from build123d import *

# Parameters (mm, degrees)
BOSS_EXTRUDE1_DEPTH     = 25.4
CUT_EXTRUDE1_DEPTH      = 58.783799795
CUT_EXTRUDE1_DEPTH_BACK = 58.783799795
SKETCH2_R               = 6.35


with BuildPart() as part:
    # Sketch1 → Boss-Extrude1 (new, symmetric)
    with BuildSketch(Plane.XY):
        Polygon((-25.4, 0), (25.4, 0), (32.118057965, 38.1), (35.244822581, 37.548667036), (28.064141329, -3.175), (-28.064141329, -3.175), (-35.244822581, 37.548667036), (-32.118057965, 38.1), align=None)
    extrude(amount=BOSS_EXTRUDE1_DEPTH, both=True)

    # Sketch2 → Cut-Extrude1 (cut, two sides: drawn at the far end of the back side and taken through both)
    with BuildSketch(Plane(origin=(0, 0, 0), x_dir=(0, 0, -1), z_dir=(1, 0, 0)).offset(-CUT_EXTRUDE1_DEPTH_BACK)):
        with Locations(Location((0, 25.4, 0), (0, 0, 90))):
            Circle(SKETCH2_R)
    extrude(amount=CUT_EXTRUDE1_DEPTH + CUT_EXTRUDE1_DEPTH_BACK, mode=Mode.SUBTRACT)


solid = part.part
Source: CAD feature listing. Evaluate the final solid. Frame: model axes, mm. A direction names the side the tool comes from. Give positions to 0.01 mm unless a question says otherwise; leave off trailing zeros. Write each loop counter-clockwise with the first axis right and the second up, starting at its lowest first coordinate (ties: lowest second). Pieces come first, ordered by that corner, then holes. Notation, with made-up numbers: M 81.5,-6 L 125.5,-6 A17 ccw 125.5,23 Z; hole C 29,39.25 d1. An arc over 180 degrees is marked long. Answer as a JSON object with one key per item and string values.
Q1. Contact query for flat-ended pins moving along their axis: P1, Ø5, axis at y = 11, z = 13.5, coming from the -X side; P2, Ø1, axis at y = 22, z = -10.5, coming from the +X side; P3, Ø16.5, axis at y = 25.4, z = 0, coming from the +X side. Output: stop coordinate, or through.
Geometry check:
{"P1": "stops at x = -31", "P2": "stops at x = 32.59", "P3": "stops at x = 34.56"}
Q2. Cut plane D-D, the plane y = 15. Return the cut outline in (x, z).
Geometry check:
{"outline": "M -31.27,-25.4 L -28.04,-25.4 L -28.04,25.4 L -31.27,25.4 Z; M 28.04,-25.4 L 31.27,-25.4 L 31.27,25.4 L 28.04,25.4 Z"}
Q3. Cut plane C-C, the plane z = 0. Return the cut outline in (x, y) (3 decimals).
Geometry check:
{"outline": "M -35.245,37.549 L -34.222,31.75 L -30.998,31.75 L -32.118,38.1 Z; M -31.983,19.05 L -28.064,-3.175 L 28.064,-3.175 L 31.983,19.05 L 28.759,19.05 L 25.4,0 L -25.4,0 L -28.759,19.05 Z; M 30.998,31.75 L 34.222,31.75 L 35.245,37.549 L 32.118,38.1 Z"}
Q4. Cut plane A-A, the plane z = 9. Return the cut outline in (x, y) (3 decimals), then the cut area to 3 significant figures.
Geometry check:
{"outline": "M -35.245,37.549 L -28.064,-3.175 L 28.064,-3.175 L 35.245,37.549 L 32.118,38.1 L 25.4,0 L -25.4,0 L -32.118,38.1 Z", "area": "424 mm^2"}
Q5. Access query for faces 4 (the face through (0, -1, -25.4)), 5 (the face through (-28.06, 15.08, 0.36)). Directions: +Z, -Z, +X, -X, +Y, -Y. A direction counts if a zero-diameter tool reaches every point of the face in a straight line with its end or side. Return the directions, or none.
Geometry check:
{"face 4": "-Z, +X, -X, +Y, -Y", "face 5": "+Z, -Z, +Y"}
Q6. Cut plane B-B, the plane y = 25.4. Return the cut outline in (x, z), then the cut area to 3 significant figures.
Geometry check:
{"outline": "M -33.1,-25.4 L -29.88,-25.4 L -29.88,-6.35 L -33.1,-6.35 Z; M -33.1,6.35 L -29.88,6.35 L -29.88,25.4 L -33.1,25.4 Z; M 29.88,-25.4 L 33.1,-25.4 L 33.1,-6.35 L 29.88,-6.35 Z; M 29.88,6.35 L 33.1,6.35 L 33.1,25.4 L 29.88,25.4 Z", "area": "246 mm^2"}
Q7. Mould query, pull axis X, two halves, no side actions, for faces 1 (the face through (0, 0, 0)), 2 (the face through (33.66, 37.83, 0.36)), 3 (the face through (-33.7, 37.82, 0.36)). Classes: +X half, -X half, draft (parallel to the pull), parting line (faces both ways), or undercut.
Geometry check:
{"face 1": "undercut", "face 2": "+X half", "face 3": "-X half"}
Q8. Ray query, line 1 along Z through (x, y) = (30, 25); line 2 along X through (y, z) = (34, -7.5); line 3 along X through (y, z) = (20, 10). Return the intervals inside material, ascending.
Geometry check:
{"line 1": "z = -25.4 to -6.34, 6.34 to 25.4", "line 2": "x = -34.62 to -31.4, 31.4 to 34.62", "line 3": "x = -32.15 to -28.93, 28.93 to 32.15"}
